Job drawing, mm, ordinate dimensions from the low corner. One solid piece. A direction names the side the tool comes from. Round coordinates to 2 decimals unless told otherwise and drop trailing zeros. Loops run counter-clockwise (first coordinate to the right, second up) from the corner with the lowest first, then second, coordinate; pieces in that order, holes last.
1) 3-axis set-ups, long thin cutter, end or side, ignore diameter. For the marked faces 4, 5, 6 and 7: which of +Z, -Z, +X, -X, +Y, -Y reach the whole face in a straight line?
2) Band-saw the part on A-A, the plane y = 0.65. Write the cut outline in (x, z).
3) Drop flat-ended pins along their axis: P1, Ø3, axis at y = 1, z = 2.5, coming from the +X side; P2, Ø0.5, axis at y = 1.5, z = 11, coming from the -X side; P3, Ø1.9, axis at y = 1, z = 11, coming from the +X side. Give the stop position or say it passes through.
4) Probe line 1 (X direction, y = 3.5, z = 11.65); line 2 (Y direction, x = 4.5, z = 11.1); line 3 (Z direction, x = 5, y = 2.7). List the from-to ranges inside material, lowest first.
5) Band-saw the part on D-D, the plane y = 1.85. Write the cut outline in (x, z).
6) Band-saw the part on C-C, the plane z = 6. Write the cut outline in (x, y), then the cut area to 3 significant figures.
7) Mould opens along X. For the marked faces 1, 2 and 3 say: +X half, -X half, draft (parallel to the pull), parting line (faces both ways), or undercut.
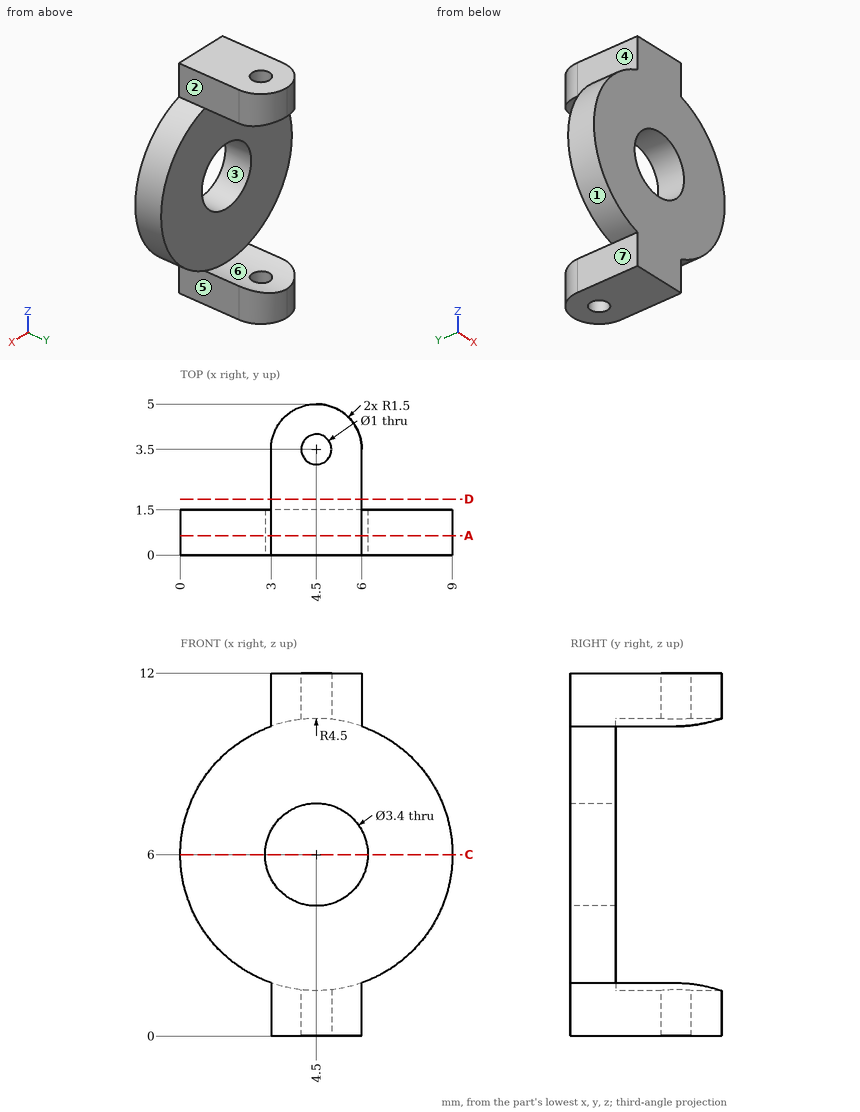
Reported:
1. face 4: +Z, -X, +Y, -Y
1. face 5: -Z, +X, +Y, -Y
1. face 6: +Y
1. face 7: -Z, -X, +Y, -Y
2. outline: (3, 0) - (6, 0) - (6, 1.76) arc R4.5 ccw to (6, 10.24) - (6, 12) - (3, 12) - (3, 10.24) arc R4.5 ccw to (3, 1.76) - close; hole circle Ø3.4 at (4.5, 6)
3. P1: stops at x = 8.53
3. P2: stops at x = 3
3. P3: stops at x = 6.46
4. line 1: x = 3 to 4, 5 to 6
4. line 2: y = 0 to 3, 4 to 5
4. line 3: z = 0 to 1.53, 10.47 to 12
5. outline: (3, 0) - (6, 0) - (6, 1.76) arc R4.5 cw to (3, 1.76) - close; (3, 10.24) arc R4.5 cw to (6, 10.24) - (6, 12) - (3, 12) - close
6. outline: (0, 0) - (2.8, 0) - (2.8, 1.5) - (0, 1.5) - close; (6.2, 0) - (9, 0) - (9, 1.5) - (6.2, 1.5) - close
6. area: 8.40 mm2
7. face 1: -X half
7. face 2: +X half
7. face 3: undercut
